```python
from build123d import *

# Parameters (mm, degrees)
BOSS_EXTRUDE1_DEPTH = 3.125
EDGE_FLANGE1_DEPTH  = 13
FILLET1_R           = 3.175
SKETCH10_R          = 1.5875
CUT_EXTRUDE1_DEPTH  = 10
LPATTERN1_COUNT     = 6
LPATTERN1_PITCH     = 24.6
SKETCH13_R          = 1.05
CUT_EXTRUDE2_DEPTH  = 10


# Sheet-metal steps are written as plain solids
with BuildPart() as part:
    # Sketch1 → Boss-Extrude1 (new body)
    with BuildSketch(Plane.XY):
        with BuildLine():
            Line((123482.998157255, 24999.885796135), (123482.998157255, 25132.885796135))
            ThreePointArc((123482.998157255, 25132.885796135), (123482.99666513, 25133.030321276), (123482.992189393, 25133.174784804))
            ThreePointArc((123482.992189393, 25133.174784804), (123480.844655225, 25137.936682931), (123475.998158089, 25139.885796135))
            Line((123475.998158089, 25139.885796135), (123469.998184079, 25139.88579685))
            ThreePointArc((123469.998184079, 25139.88579685), (123459.391582886, 25144.279196396), (123454.998185868, 25154.885798636))
            Line((123454.998185868, 25154.885798636), (123454.998186963, 25164.077536847))
            ThreePointArc((123454.998186963, 25164.077536847), (123454.412390106, 25165.491761067), (123452.998157255, 25166.077537085))
            Line((123452.998157255, 25166.077537085), (123452.998157255, 25179.077537085))
            ThreePointArc((123452.998157255, 25179.077537085), (123463.604778809, 25174.684148675), (123467.998186963, 25164.077535299))
            Line((123467.998186963, 25164.077535299), (123467.998185868, 25154.885797087))
            ThreePointArc((123467.998185868, 25154.885797087), (123468.583972137, 25153.471583456), (123469.998185629, 25152.88579685))
            Line((123469.998185629, 25152.88579685), (123475.998159637, 25152.885796136))
            ThreePointArc((123475.998159637, 25152.885796136), (123490.140293721, 25147.027930917), (123495.998157255, 25132.885796135))
            Line((123495.998157255, 25132.885796135), (123495.998157255, 25003.060796135))
            ThreePointArc((123495.998157255, 25003.060796135), (123495.068221285, 25000.815732105), (123492.823157255, 24999.885796135))
            Line((123492.823157255, 24999.885796135), (123482.998157255, 24999.885796135))
        make_face()
    extrude(amount=BOSS_EXTRUDE1_DEPTH)

    # Edge-Flange1 section (across the edge) → Edge-Flange1 (add)
    with BuildSketch(Plane(origin=(123449.873157255, 25179.077537085, 3.125), x_dir=(1, 0, 0), z_dir=(0, -1, 0))):
        with BuildLine():
            Line((-3.125, 3.125), (-3.125, 41.875))
            Line((-3.125, 41.875), (0, 41.875))
            Line((0, 41.875), (0, 3.125))
            ThreePointArc((0, 3.125), (0.915291309, 0.915291309), (3.125, 0))
            Line((3.125, 0), (3.125, -3.125))
            ThreePointArc((3.125, -3.125), (-1.294417382, -1.294417382), (-3.125, 3.125))
        make_face()
    extrude(amount=EDGE_FLANGE1_DEPTH)

    # Fillet1
    fillet1_edges = [part.edges().sort_by_distance(p)[0] for p in [
        (123482.998157255, 24999.885796135, 1.5625),
        (123448.310657255, 25179.077537085, 45),
        (123448.310657255, 25166.077537085, 45),
    ]]
    fillet(fillet1_edges, radius=FILLET1_R)

    # Sketch10 → Cut-Extrude1 (cut)
    with BuildSketch(Plane.XY.offset(3.125)):
        with Locations((123491.798157255, 25005.027537086)):
            Circle(SKETCH10_R)
    cut_extrude1 = extrude(amount=-CUT_EXTRUDE1_DEPTH, mode=Mode.SUBTRACT)

    # LPattern1: Cut-Extrude1 ×6
    with Locations(*[(0, i * LPATTERN1_PITCH, 0) for i in range(1, LPATTERN1_COUNT)]):
        add(cut_extrude1, mode=Mode.SUBTRACT)

    # Sketch13 → Cut-Extrude2 (cut)
    with BuildSketch(Plane(origin=(0, 0, 0), x_dir=(-1, 0, 0), z_dir=(0, 0, -1))):
        with Locations((-123459.498186107, 25156.8857981)):
            Circle(SKETCH13_R)
    extrude(amount=-CUT_EXTRUDE2_DEPTH, mode=Mode.SUBTRACT)


solid = part.part
```
The listing builds one solid part. Answer for the finished solid, in the listing's coordinates (mm). A direction names the side the tool comes from. Give positions to 0.01 mm unless a question says otherwise; leave off trailing zeros. Write each loop counter-clockwise with the first axis right and the second up, starting at its lowest first coordinate (ties: lowest second). Pieces come first, ordered by that corner, then holes. Notation, with made-up numbers: (72.5, 72.5) -> (86.5, 72.5) arc R24 ccw to (86.5, 85.5) -> close; hole circle Ø11 at (23.25, 58). An arc over 180 degrees is marked (long way). Write item = value, one per line. Start each with the question number.
1) Straight lines are drawn through the part: line 1 along Z through (x, y) = (123471.5, 25149) (3 decimals); line 2 along X through (y, z) = (25167, 33.5). For each, find the intervals that lie inside material, in ascending order.
2) Determine the mould class of faces 1 (the face through (123449, 25166.078, 21)), 2 (the face through (123467.998, 25160, 2)), 3 (the face through (123493.312, 25103.904, 1.584)) for opening direction Y: +Y half, -Y half, draft (parallel to the pull), parting line (faces both ways), or undercut.
3) The part is cut by section A-A, the plane y = 25107.5. Determine the outline of the cut face in (x, z) (3 decimals).
4) The part is cut by section B-B, the plane x = 123478.5. Determine the outline of the cut face in (y, z) (3 decimals).
5) Which of the six approach directions +Z, -Z, +X, -X, +Y, -Y give full straight-line access (tool end or side, diameter ignored) to faces 4 (the face through (123448.63, 25172.67, 1.78)), 5 (the face through (123473, 25152.886, 2)), 6 (the face through (123482.998, 25067, 2)), 7 (the face through (123449.873, 25173, 26))?
6) Each of these flat-tipped pins is pushed along its axis until it touches: pin 1 (8 mm diameter, centred on y = 25137.5, z = 11, fed in from +X); pin 2 (8 mm diameter, centred on x = 123461, y = 25156, fed in from +Z) (3 decimals); pin 3 (10.5 mm diameter, centred on y = 25174, z = 21.5, fed in from +X); pin 4 (0.9 mm diameter, centred on y = 25159, z = 2, fed in from -X). Where does it stop, or does it pass through?
Solutions:
q1.line_1 = 0 to 3.125
q1.line_2 = 123446.75 to 123449.87
q2.face_1 = -Y half
q2.face_2 = draft
q2.face_3 = undercut
q3.outline = (123482.998, 0) -> (123495.998, 0) -> (123495.998, 3.125) -> (123482.998, 3.125) -> close
q4.outline = (25139.423, 0) -> (25152.729, 0) -> (25152.729, 3.125) -> (25139.423, 3.125) -> close
q5.face_4 = -Z, -X, +Y, -Y
q5.face_5 = +Z, -Z, +X, +Y
q5.face_6 = +Z, -Z, -X, -Y
q5.face_7 = +Z, +X, +Y, -Y
q6.pin_1 = through
q6.pin_2 = 3.125
q6.pin_3 = 123449.87
q6.pin_4 = 123455
